Can you work these out from the model? Positions are in its coordinate system, mm. A direction names the side the tool comes from. Give positions to 0.01 mm unless a question says otherwise; leave off trailing zeros. Order: outer loops, then holes, each group sorted by start corner. A loop starts at its lowest first (then second) coordinate and runs counter-clockwise, first axis right, second up.
Item 1: I want a section at B-B, the plane z = 0. Write out the boundary of the cut face in (x, y).
Item 2: If I drill on line 1 along Z through (x, y) = (0, 5.6); line 2 along X through (y, z) = (1.75, 11.5); line 3 along Z through (x, y) = (16.5, 1.25), over which ranges is the centre line in solid material (lowest first)?
Item 3: I want a section at C-C, the plane y = 1. Write out the boundary of the cut face in (x, z), then the cut area to 3 significant figures.
Item 4: Which directions (+Z, -Z, +X, -X, +Y, -Y) give clear straight access to the entire face, cutting with the end or side of a thin tool? Please do faces 1 (the flat face through (-2.756, 2, -13)), 2 (the flat face through (-9, 0, -9)).
Item 5: If we mould it in two halves opening along X, with no side actions, what happens to faces 3 (the flat face through (2.756, 2, -13)), 4 (the flat face through (-17.76, 3.13, 17.8)), 5 (the flat face through (19.05, 3, 0))? For each: +X half, -X half, draft (parallel to the pull), parting line (faces both ways), or undercut.
Item 6: I'm going to push a flat-ended pin straight in: pin 1 Ø1.7 at (x, z) = (-13.5, 1) entering from -Y. Where does the tip first touch, or does it pass through?
Item 7: I want a section at A-A, the plane x = 0. Write out the boundary of the cut face in (y, z).
Item 8: I want a section at D-D, the plane y = 4.5. Count the separate pieces of the cut face and the enclosed holes in it, then the cut area to 3 significant figures.
```python
from build123d import *

# Parameters (mm, degrees)
SKETCH1_W           = 38.1
SKETCH1_H           = 38.1
SKETCH1_R           = 11.43
BOSS_EXTRUDE1_DEPTH = 6.35
SKETCH2_R           = 1.6002
SKETCH2_R_2         = 1.4351
CUT_EXTRUDE1_DEPTH  = 7.35
CIRPATTERN1_COUNT   = 4
CHAMFER1_SIZE       = 2.54
CUT_EXTRUDE2_DEPTH  = 3.7592
CIRPATTERN4_COUNT   = 4


with BuildPart() as part:
    # Sketch1 → Boss-Extrude1 (new body)
    with BuildSketch(Plane(origin=(0, 0, 0), x_dir=(1, 0, 0), z_dir=(0, 1, 0))):
        Rectangle(SKETCH1_W, SKETCH1_H)
        Circle(SKETCH1_R, mode=Mode.SUBTRACT)
    extrude(amount=BOSS_EXTRUDE1_DEPTH)

    # Sketch2 → Cut-Extrude1 (cut, through all)
    with BuildSketch(Plane(origin=(0, 6.35, 0), x_dir=(1, 0, 0), z_dir=(0, 1, 0))):
        with Locations((0, 13.9954)):
            Circle(SKETCH2_R)
        with Locations((15.24, 15.24)):
            Circle(SKETCH2_R_2)
    cut_extrude1 = extrude(amount=-CUT_EXTRUDE1_DEPTH, mode=Mode.SUBTRACT)

    # CirPattern1: Cut-Extrude1 ×4 about axis
    cirpattern1_axis = Axis((0, 0, 0), (0, 1, 0))
    for i in range(1, CIRPATTERN1_COUNT):
        add(cut_extrude1.rotate(cirpattern1_axis, i * 360 / CIRPATTERN1_COUNT), mode=Mode.SUBTRACT)

    # Chamfer1
    chamfer1_edges = [part.edges().sort_by_distance(p)[0] for p in [
        (19.05, 3.175, 19.05),
        (-19.05, 3.175, 19.05),
        (-19.05, 3.175, -19.05),
        (19.05, 3.175, -19.05),
    ]]
    chamfer(chamfer1_edges, length=CHAMFER1_SIZE)

    # Sketch3 → Cut-Extrude2 (cut)
    with BuildSketch(Plane.XZ):
        with BuildLine():
            Line((2.7559, 13.9954), (2.7559, 0))
            ThreePointArc((2.7559, 0), (0, -2.7559), (-2.7559, 0))
            Line((-2.7559, 0), (-2.7559, 13.9954))
            ThreePointArc((-2.7559, 13.9954), (0, 16.7513), (2.7559, 13.9954))
        make_face()
    cut_extrude2 = extrude(amount=-CUT_EXTRUDE2_DEPTH, mode=Mode.SUBTRACT)

    # CirPattern4: Cut-Extrude2 ×4 about axis
    cirpattern4_axis = Axis((0, 0, 0), (0, 1, 0))
    for i in range(1, CIRPATTERN4_COUNT):
        add(cut_extrude2.rotate(cirpattern4_axis, i * 360 / CIRPATTERN4_COUNT), mode=Mode.SUBTRACT)


solid = part.part
```
Results list:
1. outline: (-19.05, 0) - (-16.75, 0) - (-16.75, 3.76) - (-15.6, 3.76) - (-15.6, 6.35) - (-19.05, 6.35) - close; (-12.4, 3.76) - (-11.43, 3.76) - (-11.43, 6.35) - (-12.4, 6.35) - close; (11.43, 3.76) - (12.4, 3.76) - (12.4, 6.35) - (11.43, 6.35) - close; (15.6, 3.76) - (16.75, 3.76) - (16.75, 0) - (19.05, 0) - (19.05, 6.35) - (15.6, 6.35) - close
2. line 1: z = -19.05 to -15.6, -12.4 to -11.43, 11.43 to 12.4, 15.6 to 19.05
2. line 2: x = -19.05 to -2.76, 2.76 to 19.05
2. line 3: z = -19.05 to -15.93, -14.55 to -1.15, 1.15 to 14.55, 15.93 to 19.05
3. outline: (-19.05, -16.51) - (-16.51, -19.05) - (16.51, -19.05) - (19.05, -16.51) - (19.05, 16.51) - (16.51, 19.05) - (-16.51, 19.05) - (-19.05, 16.51) - close; hole circle Ø2.87 at (-15.24, -15.24); hole circle Ø2.87 at (-15.24, 15.24); hole (-14, -2.76) - (-11.09, -2.76) arc R11.43 ccw to (-2.76, -11.09) - (-2.76, -14) arc R2.76 ccw to (2.76, -14) - (2.76, -11.09) arc R11.43 ccw to (11.09, -2.76) - (14, -2.76) arc R2.76 ccw to (14, 2.76) - (11.09, 2.76) arc R11.43 ccw to (2.76, 11.09) - (2.76, 14) arc R2.76 ccw to (-2.76, 14) - (-2.76, 11.09) arc R11.43 ccw to (-11.09, 2.76) - (-14, 2.76) arc R2.76 ccw to start; hole circle Ø2.87 at (15.24, -15.24); hole circle Ø2.87 at (15.24, 15.24)
3. area: 896 mm2
4. face 1: -Y
4. face 2: +Z, -Z, +X, -X, -Y
5. face 3: undercut
5. face 4: -X half
5. face 5: +X half
6. pin 1: stops at y = 3.76
7. outline: (0, -19.05) - (6.35, -19.05) - (6.35, -15.6) - (3.76, -15.6) - (3.76, -16.75) - (0, -16.75) - close; (0, 16.75) - (3.76, 16.75) - (3.76, 15.6) - (6.35, 15.6) - (6.35, 19.05) - (0, 19.05) - close; (3.76, -12.4) - (6.35, -12.4) - (6.35, -11.43) - (3.76, -11.43) - close; (3.76, 11.43) - (6.35, 11.43) - (6.35, 12.4) - (3.76, 12.4) - close
8. separate pieces: 1
8. enclosed holes: 9
8. area: 970 mm2
